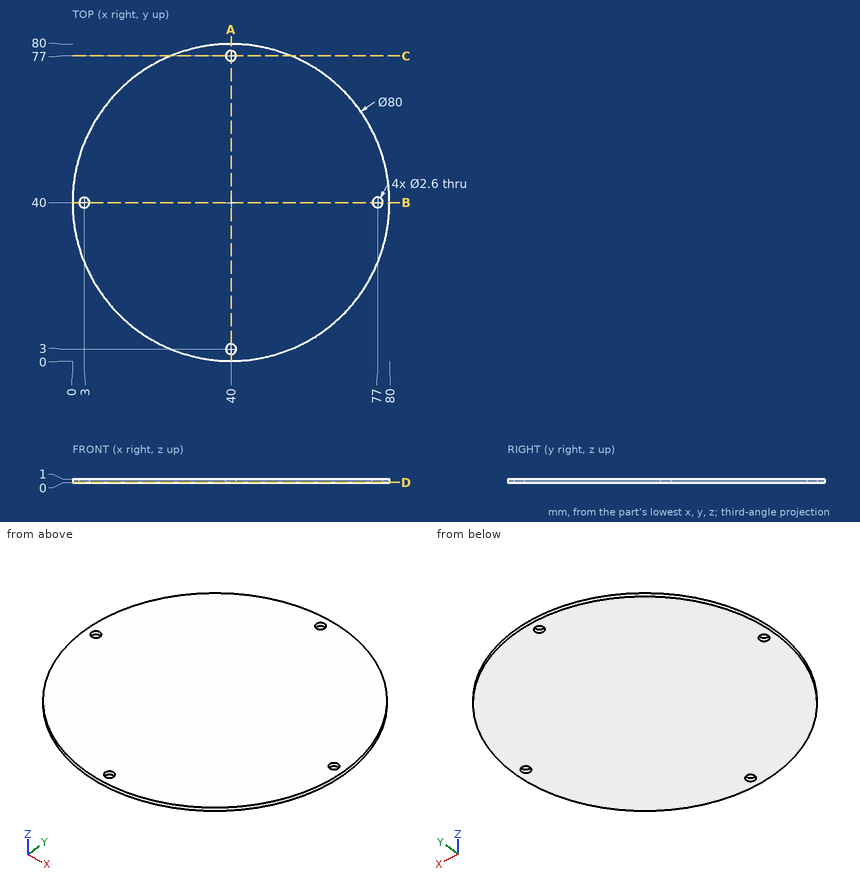
Study the drawing (mm; zero at the part's minimum x, y, z) and answer. Round coordinates to 2 decimals unless told otherwise and drop trailing zeros. Write each loop counter-clockwise with the first axis right and the second up, starting at its lowest first coordinate (ties: lowest second). Pieces come first, ordered by that corner, then holes.
1) A cutting plane is placed at A-A (x = 40). Give the vertices of the cut face in (y, z), plus the area to 3 significant figures.
2) Straight lines are drawn through the part: line 1 (Y direction, x = 40, z = 0.6); line 2 (Y direction, x = 3, z = 0.6). For each, find the intervals that lie inside material, in ascending order.
3) A cutting plane is placed at C-C (y = 77). Give the vertices of the cut face in (x, z), plus the area to 3 significant figures.
4) A cutting plane is placed at D-D (z = 0.15). Give the vertices of the cut face in (x, y), plus the area to 3 significant figures.
5) Given pin 1 Ø2.5 at (x, y) = (40, 3) entering from -Z, flat-ended and moving along its own axis, determine where the tip first touches the part or whether it passes through.
Completed:
1. outline: (0, 0) - (1.7, 0) - (1.7, 1) - (0, 1) - close; (4.3, 0) - (75.7, 0) - (75.7, 1) - (4.3, 1) - close; (78.3, 0) - (80, 0) - (80, 1) - (78.3, 1) - close
1. area: 74.8 mm2
2. line 1: y = 0 to 1.7, 4.3 to 75.7, 78.3 to 80
2. line 2: y = 24.8 to 38.7, 41.3 to 55.2
3. outline: (24.8, 0) - (38.7, 0) - (38.7, 1) - (24.8, 1) - close; (41.3, 0) - (55.2, 0) - (55.2, 1) - (41.3, 1) - close
3. area: 27.8 mm2
4. outline: circle Ø80 at (40, 40); hole circle Ø2.6 at (3, 40); hole circle Ø2.6 at (40, 3); hole circle Ø2.6 at (40, 77); hole circle Ø2.6 at (77, 40)
4. area: 5,010 mm2
5. pin 1: passes through
